Print and shaded views of the part. All mm, measured from the part's lowest x, y and z. Coordinates: 2 decimals unless noted, no trailing zeros. Loops run counter-clockwise (first coordinate to the right, second up) from the corner with the lowest first, then second, coordinate; pieces in that order, holes last. Notation, with made-up numbers: (14, -3.75) -> (69, -3.75) arc R25 ccw to (69, 28.25) -> close; hole circle Ø5 at (62.25, 83.25). An arc over 180 degrees is marked (long way). One line per question, with ' | ' between items. Start each with the question number.
1) Cut at A-A (x = 36). List the corners of the cut face in (y, z).
2) Cut at C-C (z = 25). List the corners of the cut face in (x, y).
3) Cut at B-B (y = 31). List the corners of the cut face in (x, z), plus the area to 3 significant figures.
4) Probe L1, parallel to Z at x = 31, y = 33.5; L2, parallel to Y at x = 19, z = 24; L3, parallel to Y at x = 14, z = 22. List the from-to ranges inside material, lowest first. Write a range as from..to.
5) Drop flat-ended pins along their axis: pin 1 (4 mm diameter, centred on x = 18.5, z = 22.5, fed in from +Y); pin 2 (2 mm diameter, centred on y = 15, z = 12, fed in from -X); pin 3 (3 mm diameter, centred on x = 28.5, z = 22.5, fed in from +Y). Give the stop position or say it passes through.
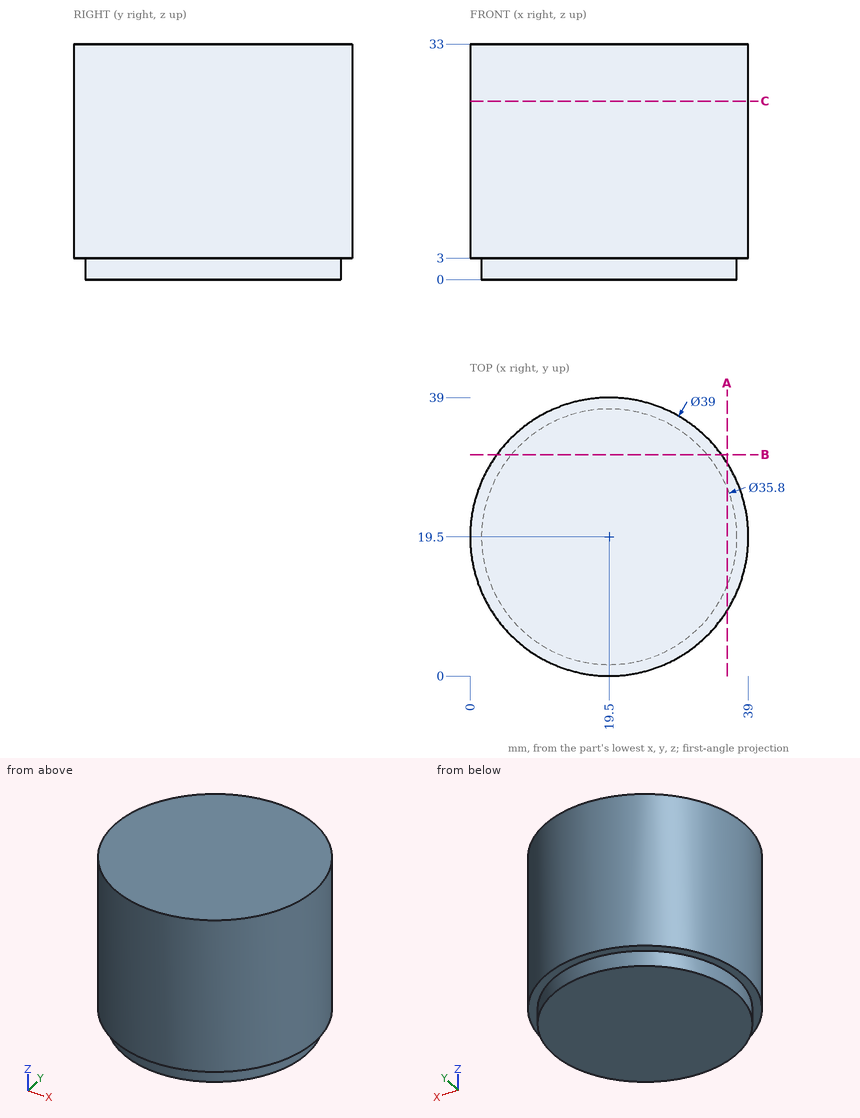
Reported:
1) outline: (9.11, 3) -> (12.56, 3) -> (12.56, 0) -> (26.44, 0) -> (26.44, 3) -> (29.89, 3) -> (29.89, 33) -> (9.11, 33) -> close
2) outline: circle Ø39 at (19.5, 19.5)
3) outline: (3.75, 3) -> (5.78, 3) -> (5.78, 0) -> (33.22, 0) -> (33.22, 3) -> (35.25, 3) -> (35.25, 33) -> (3.75, 33) -> close | area: 1,030 mm²
4) L1: z = 3..33 | L2: y = 0.01..38.99 | L3: y = 0.79..38.21
5) pin 1: stops at y = 39 | pin 2: stops at x = 0.32 | pin 3: stops at y = 37.5
